The model under review builds one solid part; all positions refer to its coordinate system, in mm. Coordinates: 2 decimals unless noted, no trailing zeros. Order: outer loops, then holes, each group sorted by start corner. A loop starts at its lowest first (then second) coordinate and runs counter-clockwise, first axis right, second up. Notation, with made-up numbers: M 17,-34 L 50,-34 A28 ccw 50,-8 Z; hole C 36.25,10.25 d9. An arc over 180 degrees is marked long. Answer in a Markdown table with one row per item.
Autodesk Inventor part; units mm, degrees
ref_plane "M_XY" through (0, 0, 0) normal (1, 0, 0) x (0, 0, -1)
ref_plane "M_YZ" through (0, 0, 0) normal (0, 0, -1) x (0, 1, 0)
ref_plane "M_ZX" through (0, 0, 0) normal (0, 1, 0) x (1, 0, 0)
sketch "Skizze_1" plane through (0, 0, 0) normal (0, 1, 0) x (-1, 0, 0)
  line L0 (-3.749, 0) -> (-1.549, 0)
  line L1 (-1.549, 0) -> (-1.549, -3.5)
  line L2 (-1.549, -3.5) -> (-2.649, -7.6053)
  line L3 (-2.649, -7.6053) -> (-3.749, -3.5)
  line L4 (-3.749, -3.5) -> (-3.749, 0)
  line L5 (-3.749, 0) -> (-1.549, 0)
revolve "Revolution1" add sketch "Skizze_1" angle 360 about axis through (3.749, 0, 0) along (1, 0, 0)
sketch "Skizze_2" plane through (0, 0, 0) normal (1, 0, 0) x (0, 1, 0)
  line L0 (-35, 26) -> (-35, -52)
  line L1 (-35, -52) -> (26, -52)
  line L2 (26, -52) -> (26, 26)
  line L3 (26, 26) -> (-35, 26)
  line L4 (-2.0207, 3.5) -> (-4.0415, 0)
  line L5 (-4.0415, 0) -> (-2.0207, -3.5)
  line L6 (-2.0207, -3.5) -> (2.0207, -3.5)
  line L7 (2.0207, -3.5) -> (4.0415, 0)
  line L8 (4.0415, 0) -> (2.0207, 3.5)
  line L9 (2.0207, 3.5) -> (-2.0207, 3.5)
extrude "Extrusion1" cut sketch "Skizze_2" along normal blind 10
sketch "Skizze_3" plane through (0, 0, 0) normal (0, 1, 0) x (-1, 0, 0)
  line L0 (-3.749, 0) -> (-1.549, 0)
  line L1 (-1.549, 0) -> (-1.549, -2)
  line L2 (-1.549, -2) -> (-1.928, -1.621)
  line L3 (-1.928, -1.621) -> (-3.37, -1.621)
  line L4 (-3.37, -1.621) -> (-3.749, -2)
  line L5 (-3.749, -2) -> (-3.749, 0)
  line L6 (-3.749, 0) -> (-1.549, 0)
revolve "Revolution2" cut sketch "Skizze_3" angle 360 about axis through (3.749, 0, 0) along (1, 0, 0)
thread "Thread1"
ref_plane "M_XY" through (0, 0, 0) normal (1, 0, 0) x (0, 0, -1)
ref_plane "M_YZ" through (0, 0, 0) normal (0, 0, -1) x (0, 1, 0)
ref_plane "M_ZX" through (0, 0, 0) normal (0, 1, 0) x (1, 0, 0)
properties part number "205-S-M"
(1) Take a section at A-A (x = 2.7). Write out the cut boundary in (y, z), then the cut area to 3 significant figures.
Report:
| item | result |
|---|---|
| outline | M -4.04,0 L -2.02,-3.5 L 2.02,-3.5 L 4.04,0 L 2.02,3.5 L -2.02,3.5 Z; hole C 0,0 d3.24 |
| area | 34.2 mm^2 |
(2) To check wall thickness, follow line 1 (Y direction, x = 3, z = -0.5); line 2 (Z direction, x = 3.05, y = 1); line 3 (Z direction, x = 1.65, y = -1.25). State the ranges of each line that lie inside material, in increasing order. Write a range as [from, to].
Report:
| item | result |
|---|---|
| line 1 | [-3.75, -1.54], [1.54, 3.75] |
| line 2 | [-3.5, -1.28], [1.28, 3.5] |
| line 3 | [-3.5, -1.43], [1.43, 3.5] |
(3) The part is to be moulded in two halves that separate along Z. For faces 1 (the cylindrical face through (2.659, -1.438, -0.748)), 2 (the flat face through (3.749, -2, -2)), 3 (the flat face through (2.634, -3.045, -1.726)), 4 (the conical face through (3.71, 3.65, 0.08)), say which applies: +Z half, -Z half, draft (parallel to the pull), parting line (faces both ways), or undercut.
Report:
| item | result |
|---|---|
| face 1 | undercut |
| face 2 | draft |
| face 3 | -Z half |
| face 4 | parting line |
